```python
from build123d import *

# Parameters (mm, degrees)
SKETCH_1_W             = 40
SKETCH_1_H             = 640
EXTRUDE_1_DEPTH        = 5
SKETCH_2_R             = 3
CUT_EXTRUDE_1_DEPTH    = 321.780298647
PATTERN_LINEAR_1_COUNT = 5
PATTERN_LINEAR_1_PITCH = 150


with BuildPart() as part:
    # Эскиз1 → Бобышка-Вытянуть1 (new, symmetric)
    with BuildSketch(Plane(origin=(0, 0, 0), x_dir=(1, 0, 0), z_dir=(0, 1, 0))):
        Rectangle(SKETCH_1_W, SKETCH_1_H)
    extrude(amount=EXTRUDE_1_DEPTH, both=True)

    # Эскиз2 → Вырез-Вытянуть1 (cut, through all)
    with BuildSketch(Plane(origin=(0, 5, 0), x_dir=(1, 0, 0), z_dir=(0, 1, 0))):
        with Locations(Location((0, -300, 0), (0, 0, 270))):
            Circle(SKETCH_2_R)
    cut_extrude_1 = extrude(amount=-CUT_EXTRUDE_1_DEPTH, mode=Mode.SUBTRACT)

    # Линейный массив1: Вырез-Вытянуть1 ×5
    with Locations(*[(0, 0, -i * PATTERN_LINEAR_1_PITCH) for i in range(1, PATTERN_LINEAR_1_COUNT)]):
        add(cut_extrude_1, mode=Mode.SUBTRACT)


solid = part.part
```
Geometry: final body of the model. Coordinates: model frame, mm. Coordinates: 2 decimals unless noted, no trailing zeros. Return JSON: item names as keys, results as strings. Group by question number.
1. Pin query (flat end, axial travel): pin 1 (7 mm diameter, centred on x = 0, z = 0, fed in from -Y). Return the tip coordinate at first contact, or that it passes through.
2. Pull-direction query (Z, two-part tool) for faces 1 (the face through (0, 0, -320)), 2 (the face through (0, 0, 320)), 3 (the face through (0, -5, -4)); classes: pulls with the +Z half, pulls with the -Z half, needs draft (parallel to the pull), parting line crosses it, or undercut.
3. Material intervals for line 1 along X through (y, z) = (0.5, -300), sorted ascending. Write a range as [from, to].
Resolved:
{
 "1": {"pin 1": "stops at y = -5"},
 "2": {"face 1": "pulls with the -Z half", "face 2": "pulls with the +Z half", "face 3": "needs draft"},
 "3": {"line 1": "x = [-20, -3], [3, 20]"}
}
